Check sheet for the modelled part. Datum: model origin and axes. Units: mm. A direction names the side the tool comes from. Give positions to 0.01 mm unless a question says otherwise; leave off trailing zeros. Order: outer loops, then holes, each group sorted by start corner. A loop starts at its lowest first (then second) coordinate and runs counter-clockwise, first axis right, second up. Notation, with made-up numbers: (-24, 6) -> (-2, 6) arc R5 cw to (-2, 13) -> close; hole circle Ø9 at (-33.5, 39). An arc over 180 degrees is marked (long way). Write each question's results on one line, items separated by ' | '.
from build123d import *

# Parameters (mm, degrees)
SKETCH1_W                    = 448
SKETCH1_H                    = 248
TAO_KHOI_DEPTH               = 112
SKETCH2_W                    = 412
SKETCH2_H                    = 212
TAO_VUNG_DAT_VO_TRONG_DEPTH  = 206
TAO_LO_DI_DAY_RA_NGOAI_REACH = 526.168
SKETCH3_R                    = 10
SKETCH5_R                    = 5
TAO_LO_LAY_KHI_DEPTH         = 18


with BuildPart() as part:
    # Sketch1 → tao_khoi (new, symmetric)
    with BuildSketch(Plane.XY):
        with Locations((224, 124)):
            Rectangle(SKETCH1_W, SKETCH1_H)
    extrude(amount=TAO_KHOI_DEPTH, both=True)

    # Sketch2 → tao_vung_dat_vo_trong (cut)
    with BuildSketch(Plane.XY.offset(112)):
        with Locations((224, 124)):
            Rectangle(SKETCH2_W, SKETCH2_H)
    extrude(amount=-TAO_VUNG_DAT_VO_TRONG_DEPTH, mode=Mode.SUBTRACT)

    # Sketch3 → tao_lo_di_day_ra_ngoai (cut, up to next)
    with BuildSketch(Plane(origin=(448, 0, 0), x_dir=(0, 0, -1), z_dir=(1, 0, 0)), mode=Mode.PRIVATE) as tao_lo_di_day_ra_ngoai_sk1:
        with Locations((82, 30)):
            Circle(SKETCH3_R)
    tao_lo_di_day_ra_ngoai_tool1 = extrude(tao_lo_di_day_ra_ngoai_sk1.sketch, amount=-TAO_LO_DI_DAY_RA_NGOAI_REACH, mode=Mode.PRIVATE) & part.part
    add(tao_lo_di_day_ra_ngoai_tool1.solids().sort_by_distance((448, 30, -82))[0], mode=Mode.SUBTRACT)

    # Sketch5 → tao_lo_lay_khi (cut)
    with BuildSketch(Plane(origin=(0, 248, 0), x_dir=(1, 0, 0), z_dir=(0, 1, 0))):
        with Locations(Location((379, 13, 0), (0, 0, 270))):
            Circle(SKETCH5_R)
        with Locations(Location((379, -47, 0), (0, 0, 270))):
            Circle(SKETCH5_R)
    extrude(amount=-TAO_LO_LAY_KHI_DEPTH, mode=Mode.SUBTRACT)


solid = part.part
1. Mould release check, pull along X, two halves, no side actions. Record for faces 1 (the cylindrical face through (383.957, 239.126, -13.651)), 2 (the flat face through (0, 122, 2)), 3 (the cylindrical face through (439, 24, -74)): +X half, -X half, draft (parallel to the pull), parting line (faces both ways), or undercut.
Verdict:
face 1: undercut | face 2: -X half | face 3: draft
2. Material ranges on probe 1 along Z at (x, y) = (379, 243.5); probe 2 along Y at (x, z) = (138.5, 10.5); probe 3 along X at (y, z) = (20.5, -17.5), recorded low to high. Write a range as from..to.
Verdict:
probe 1: z = -112..-18, -8..42, 52..112 | probe 2: y = 0..18, 230..248 | probe 3: x = 0..18, 430..448
3. Access from +Z, -Z, +X, -X, +Y, -Y to the whole of each face (thin tool, end or side, straight path). Record for faces 4 (the cylindrical face through (383.957, 239.126, 46.349)), 5 (the flat face through (430, 123, 10)), 6 (the flat face through (206, 14, 112)).
Verdict:
face 4: +Y | face 5: +Z | face 6: +Z, +X, -X, +Y, -Y
4. Gauge pin test, flat end, axial feed: pin 1 Ø10 at (x, y) = (343, 44.5) entering from +Z. Record the tip position at first contact, or that the pin passes through.
Verdict:
pin 1: stops at z = -94
5. Section check A-A on y = 30. Record the cut outline in (x, z).
Verdict:
outline: (0, -112) -> (448, -112) -> (448, -92) -> (430, -92) -> (430, -94) -> (18, -94) -> (18, 112) -> (0, 112) -> close; (430, -72) -> (448, -72) -> (448, 112) -> (430, 112) -> close
6. Section check C-C on x = 379. Record the cut outline in (y, z).
Verdict:
outline: (0, -112) -> (248, -112) -> (248, -18) -> (230, -18) -> (230, -94) -> (18, -94) -> (18, 112) -> (0, 112) -> close; (230, -8) -> (248, -8) -> (248, 42) -> (230, 42) -> close; (230, 52) -> (248, 52) -> (248, 112) -> (230, 112) -> close
7. Section check B-B on z = 18.5. Record the cut outline in (x, y), then the cut area to 3 significant figures.
Verdict:
outline: (0, 0) -> (448, 0) -> (448, 248) -> (0, 248) -> close; hole (18, 18) -> (430, 18) -> (430, 230) -> (18, 230) -> close | area: 23,800 mm^2
8. Section check D-D on z = 47. Record the cut outline in (x, y), then the cut area to 3 significant figures.
Verdict:
outline: (0, 0) -> (448, 0) -> (448, 248) -> (384, 248) -> (384, 230) -> (430, 230) -> (430, 18) -> (18, 18) -> (18, 230) -> (374, 230) -> (374, 248) -> (0, 248) -> close | area: 23,600 mm^2
